Source: three-view drawing plus pictorial views. Frame: mm from the lowest corner of the part. Round coordinates to 2 decimals unless told otherwise and drop trailing zeros. Loops run counter-clockwise (first coordinate to the right, second up) from the corner with the lowest first, then second, coordinate; pieces in that order, holes last. Notation, with made-up numbers: M -8,-12 L -3,-12 A29 ccw -3,12 Z; hole C -31,-38.5 d1. An arc over 180 degrees is marked long. Answer as a JSON object with one key per item and string values.
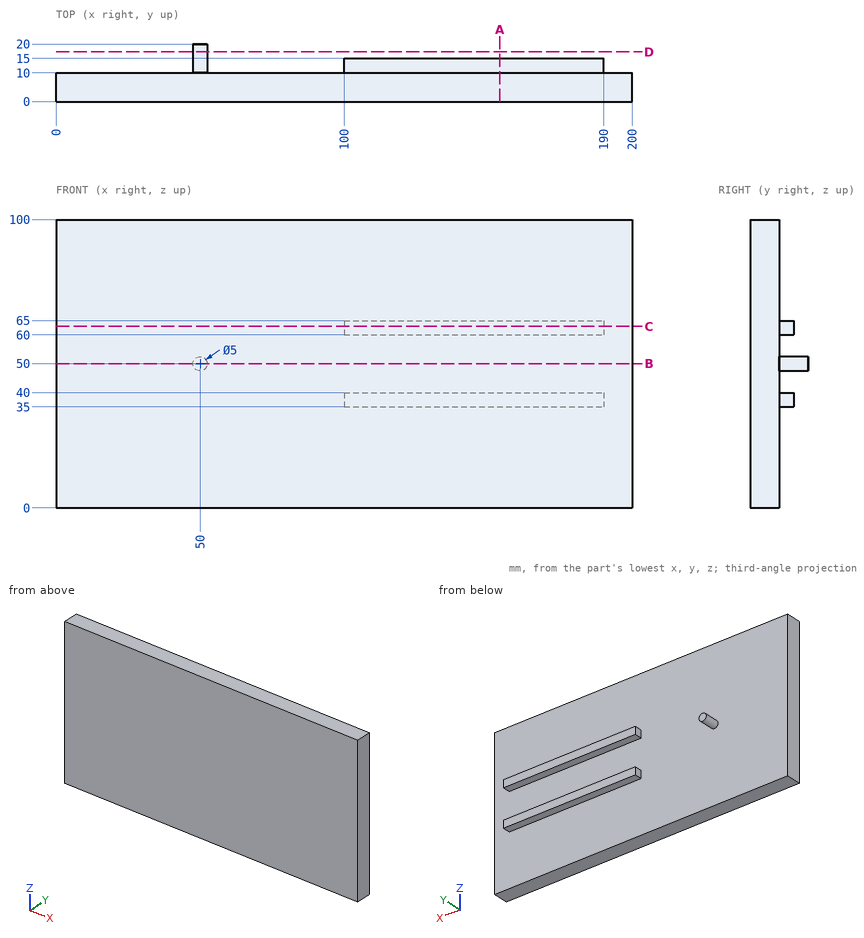
1) Cut plane D-D on y = 17.25. Return the cut outline in (x, z), and give its area (3 significant figures).
Geometry results:
{"outline": "C 50,50 d5", "area": "19.6 mm2"}
2) Cut plane B-B on z = 50. Return the cut outline in (x, y).
Geometry results:
{"outline": "M 0,0 L 200,0 L 200,10 L 52.5,10 L 52.5,20 L 47.5,20 L 47.5,10 L 0,10 Z"}
3) Cut plane C-C on z = 63. Return the cut outline in (x, y).
Geometry results:
{"outline": "M 0,0 L 200,0 L 200,10 L 190,10 L 190,15 L 100,15 L 100,10 L 0,10 Z"}
4) First-contact query: pin 1 (2.5 mm diameter, centred on x = 152.5, z = 62, fed in from +Y); pin 2 (2.5 mm diameter, centred on y = 13, z = 36.5, fed in from -X); pin 3 (2.5 mm diameter, centred on x = 158.5, y = 11.5, fed in from -Z). Flat tips, straight axial feed; report the tip coordinate or a pass-through.
Geometry results:
{"pin 1": "y = 15", "pin 2": "x = 100", "pin 3": "z = 35"}
5) Line query: probe 1 along Z at (x, y) = (179, 11.25); probe 2 along Y at (x, z) = (128, 82); probe 3 along X at (y, z) = (13.5, 36.5). Output: solid intervals per line, ascending.
Geometry results:
{"probe 1": "35 to 40, 60 to 65", "probe 2": "0 to 10", "probe 3": "100 to 190"}
6) Cut plane A-A on x = 154. Return the cut outline in (y, z), and give its area (3 significant figures).
Geometry results:
{"outline": "M 0,0 L 10,0 L 10,35 L 15,35 L 15,40 L 10,40 L 10,60 L 15,60 L 15,65 L 10,65 L 10,100 L 0,100 Z", "area": "1,050 mm2"}
